CAD build for the part. Positions are in the model's coordinates, mm. Face numbers are marked on the shaded views. A direction names the side the tool comes from. Coordinates: 2 decimals unless noted, no trailing zeros. Order: outer loops, then holes, each group sorted by start corner. A loop starts at its lowest first (then second) coordinate and runs counter-clockwise, first axis right, second up. Notation, with made-up numbers: (-21, -17.75) - (-8, -17.75) arc R18 ccw to (-8, 16.25) - close; hole circle Ø3 at (39, 26). An arc over 180 degrees is marked (long way). Use one line per item in the form item = value.
```python
from build123d import *

# Parameters (mm, degrees)
CROQUIS1_R              = 12.5
SALIENTE_EXTRUIR1_DEPTH = 64
CROQUIS2_R              = 1.5
CORTAR_EXTRUIR1_DEPTH   = 40
CROQUIS3_R              = 3.5
SALIENTE_EXTRUIR2_DEPTH = 2.5
CROQUIS4_R              = 2
SALIENTE_EXTRUIR3_DEPTH = 9.5


with BuildPart() as part:
    # Croquis1 → Saliente-Extruir1 (new body)
    with BuildSketch(Plane(origin=(0, 0, 0), x_dir=(1, 0, 0), z_dir=(0, 1, 0))):
        with Locations(Location((0, 0, 0), (0, 0, 270))):
            Circle(CROQUIS1_R)
    extrude(amount=SALIENTE_EXTRUIR1_DEPTH)

    # Croquis2 → Cortar-Extruir1 (cut)
    with BuildSketch(Plane(origin=(0, 64, 0), x_dir=(1, 0, 0), z_dir=(0, 1, 0))):
        with Locations(Location((-8.5, 0, 0), (0, 0, 270))):
            Circle(CROQUIS2_R)
        with Locations(Location((8.5, 0, 0), (0, 0, 270))):
            Circle(CROQUIS2_R)
    extrude(amount=-CORTAR_EXTRUIR1_DEPTH, mode=Mode.SUBTRACT)

    # Croquis3 → Saliente-Extruir2 (add)
    with BuildSketch(Plane(origin=(0, 64, 0), x_dir=(1, 0, 0), z_dir=(0, 1, 0))):
        with Locations(Location((0, 0, 0), (0, 0, 270))):
            Circle(CROQUIS3_R)
    extrude(amount=SALIENTE_EXTRUIR2_DEPTH)

    # Croquis4 → Saliente-Extruir3 (add)
    with BuildSketch(Plane(origin=(0, 66.5, 0), x_dir=(1, 0, 0), z_dir=(0, 1, 0))):
        with Locations(Location((0, 0, 0), (0, 0, 270))):
            Circle(CROQUIS4_R)
    extrude(amount=SALIENTE_EXTRUIR3_DEPTH)


solid = part.part
```
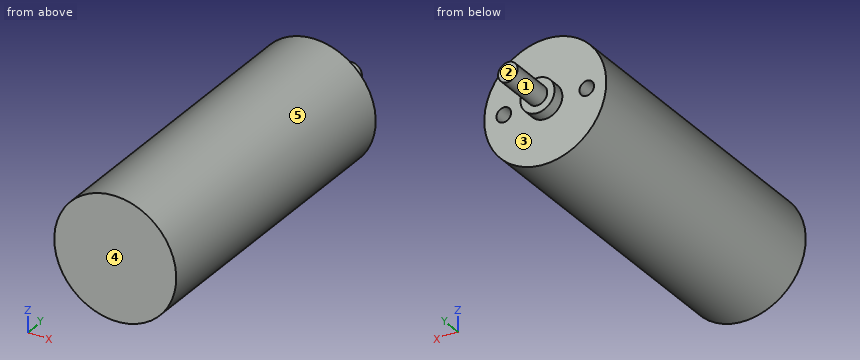
Item 1: Drill centre lines: line 1 (X direction, y = 50, z = 0); line 2 (Y direction, x = -9.75, z = 4.5); line 3 (Z direction, x = -9, y = 53.5). Where is each one in solid material? Low to high. Write a range as [from, to].
Derived:
line_1 = [-12.5, -10], [-7, 7], [10, 12.5]
line_2 = [0, 64]
line_3 = [-8.67, -1.41], [1.41, 8.67]
Item 2: Two-plate mould, pull along Y, no slides. Class the marked faces 3, 4 and 5: +Y half, -Y half, draft (parallel to the pull), parting line (faces both ways), or undercut.
Derived:
face_3 = +Y half
face_4 = -Y half
face_5 = draft
Item 3: Drop flat-ended pins along their axis: pin 1 (5 mm diameter, centred on x = -5, y = 24, fed in from -Z); pin 2 (3 mm diameter, centred on x = 8.5, z = 9, fed in from +Y); pin 3 (2.5 mm diameter, centred on x = -8.5, z = 0, fed in from -Y); pin 4 (0.9 mm diameter, centred on x = 8, z = 0.5, fed in from +Y). Give the stop position or say it passes through.
Derived:
pin_1 = -12.25
pin_2 = 64
pin_3 = 0
pin_4 = 24
Item 4: Cut at A-A, the plane x = 0. Write the cut outline in (y, z), plus the area to 3 significant figures.
Derived:
outline = (0, -12.5) - (64, -12.5) - (64, -3.5) - (66.5, -3.5) - (66.5, -2) - (76, -2) - (76, 2) - (66.5, 2) - (66.5, 3.5) - (64, 3.5) - (64, 12.5) - (0, 12.5) - close
area = 1,660 mm²
Item 5: Cut at D-D, the plane y = 16.5. Write the cut outline in (x, z), plus the area to 3 significant figures.
Derived:
outline = circle Ø25 at (0, 0)
area = 491 mm²
Item 6: 3-axis set-ups, long thin cutter, end or side, ignore diameter. For the marked faces 1 and 2: which of +Z, -Z, +X, -X, +Y, -Y reach the whole face in a straight line?
Derived:
face_1 = +Y
face_2 = +Z, -Z, +X, -X, +Y
Item 7: Cut at B-B, the plane z = 0. Write the cut outline in (x, y).
Derived:
outline = (-12.5, 0) - (12.5, 0) - (12.5, 64) - (10, 64) - (10, 24) - (7, 24) - (7, 64) - (3.5, 64) - (3.5, 66.5) - (2, 66.5) - (2, 76) - (-2, 76) - (-2, 66.5) - (-3.5, 66.5) - (-3.5, 64) - (-7, 64) - (-7, 24) - (-10, 24) - (-10, 64) - (-12.5, 64) - close
Item 8: Cut at C-C, the plane y = 30.5. Write the cut outline in (x, z), plus the area to 3 significant figures.
Derived:
outline = circle Ø25 at (0, 0); hole circle Ø3 at (-8.5, 0); hole circle Ø3 at (8.5, 0)
area = 477 mm²
